Drawing for the job (mm, zero at the part's lowest x, y, z). A direction names the side the tool comes from. Coordinates: 2 decimals unless noted, no trailing zeros. Write each loop counter-clockwise with the first axis right and the second up, starting at its lowest first coordinate (ties: lowest second). Pieces come first, ordered by that corner, then holes. Notation, with made-up numbers: M 14.25,-17.75 L 65.25,-17.75 A11 cw 65.25,2.25 Z; hole C 57,-13.75 d1. An arc over 180 degrees is marked long. Put each result on its own line as item: value. Start each with the question number.
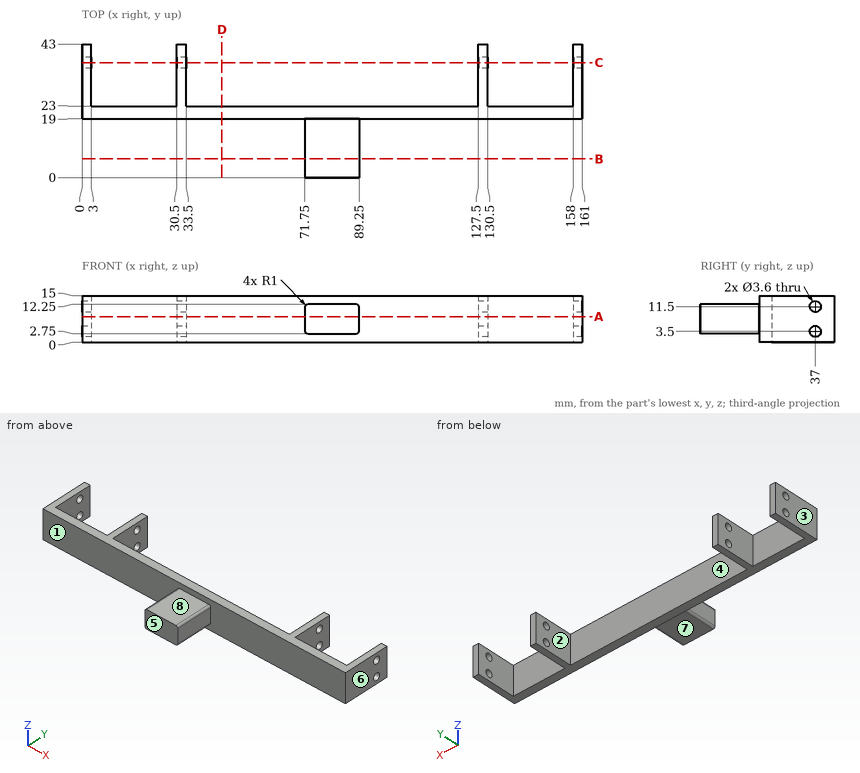
(1) Slice it at C-C, the plane y = 37. State how many separate pieces and enclosed holes the cut face has, then the cut area to 3 significant figures.
(2) Two-plate mould, pull along X, no slides. Class the marked faces 1, 2 and 3: +X half, -X half, draft (parallel to the pull), parting line (faces both ways), or undercut.
(3) Drop flat-ended pins along their axis: pin 1 (4 mm diameter, centred on y = 8.5, z = 8.5, fed in from -X); pin 2 (5 mm diameter, centred on x = 111.5, z = 13.5, fed in from +Y); pin 3 (4 mm diameter, centred on y = 8.5, z = 10, fed in from +X). Give the stop position or say it passes through.
(4) Slice it at D-D, the plane x = 45. Write the cut outline in (y, z).
(5) Slice it at A-A, the plane z = 8.25. Write the cut outline in (x, y), then the cut area to 3 significant figures.
(6) Slice it at B-B, the plane y = 6. Write the cut outline in (x, z), then the cut area to 3 significant figures.
(7) Drill centre lines: line 1 (X direction, y = 41, z = 14.25); line 2 (Y direction, x = 159.35, z = 11.5); line 3 (Y direction, x = 48, z = 9.25). Where is each one in solid material? Low to high. Write a range as [from, to].
(8) Which spindle directions (+Z, -Z, +X, -X, +Y, -Y) get a long thin tool onto all of the face, cutting with end or side? Do the marked faces 4, 5, 6, 7 and 8. Say none if no direction does.
Result set:
1. separate pieces: 12
1. enclosed holes: 0
1. area: 93.6 mm^2
2. face 1: draft
2. face 2: undercut
2. face 3: -X half
3. pin 1: stops at x = 71.75
3. pin 2: stops at y = 23
3. pin 3: stops at x = 89.25
4. outline: M 19,0 L 23,0 L 23,15 L 19,15 Z
5. outline: M 0,19 L 71.75,19 L 71.75,0 L 89.25,0 L 89.25,19 L 161,19 L 161,43 L 158,43 L 158,23 L 130.5,23 L 130.5,43 L 127.5,43 L 127.5,23 L 33.5,23 L 33.5,43 L 30.5,43 L 30.5,23 L 3,23 L 3,43 L 0,43 Z
5. area: 1,220 mm^2
6. outline: M 71.75,3.75 A1 ccw 72.75,2.75 L 88.25,2.75 A1 ccw 89.25,3.75 L 89.25,11.25 A1 ccw 88.25,12.25 L 72.75,12.25 A1 ccw 71.75,11.25 Z
6. area: 165 mm^2
7. line 1: x = [0, 3], [30.5, 33.5], [127.5, 130.5], [158, 161]
7. line 2: y = [19, 35.2], [38.8, 43]
7. line 3: y = [19, 23]
8. face 4: +Z, -Z, +Y
8. face 5: +Z, -Z, +X, -X, -Y
8. face 6: +Z, -Z, +X, +Y, -Y
8. face 7: -Z, +X, -X, -Y
8. face 8: +Z, +X, -X, -Y
